Design review of the part shown in the three views and the two pictorial views. Dimensions are in mm from the part's minimum x, y and z. Give positions to 0.01 mm unless a question says otherwise; leave off trailing zeros. Order: outer loops, then holes, each group sorted by start corner. A loop starts at its lowest first (then second) coordinate and runs counter-clockwise, first axis right, second up.
Item 1: Consider section C-C (x = 4). Give the boundary of the cut face in (y, z).
Item 2: Consider section D-D (z = 12). Give the boundary of the cut face in (x, y).
Item 3: For P1, Ø7, axis at x = 4, z = 7.5, coming from the +Y side, flat-tipped, find the tip position at first contact; note if it passes through.
Item 4: Consider section A-A (y = 0.15). Give the number of separate pieces and of enclosed holes in the cut face, plus the area to 3 significant figures.
Item 5: Consider section B-B (x = 76.5). Give the boundary of the cut face in (y, z).
Item 6: For probe 1 along X at (y, z) = (0.25, 6.75); probe 2 along X at (y, z) = (0.4, 7.5); probe 3 along Z at (x, y) = (76.5, 0.35), list the stretches that pass through material, from the lowest coordinate up.
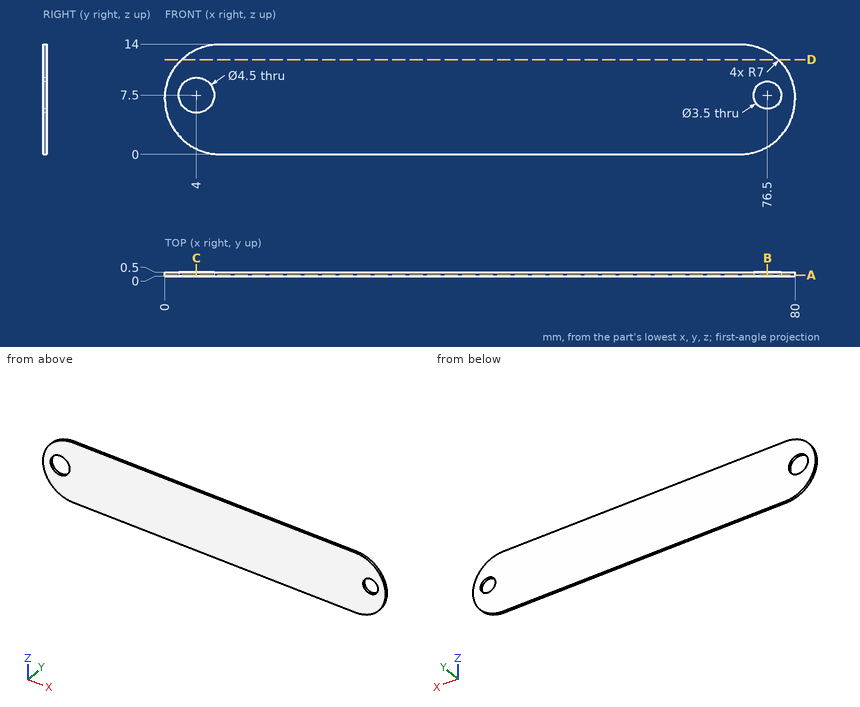
Resolved:
1. outline: (0, 0.68) - (0.5, 0.68) - (0.5, 5.25) - (0, 5.25) - close; (0, 9.75) - (0.5, 9.75) - (0.5, 13.32) - (0, 13.32) - close
2. outline: (2.1, 0) - (77.9, 0) - (77.9, 0.5) - (2.1, 0.5) - close
3. P1: stops at y = 0.5
4. separate pieces: 1
4. enclosed holes: 2
4. area: 1,050 mm2
5. outline: (0, 0.94) - (0.5, 0.94) - (0.5, 5.75) - (0, 5.75) - close; (0, 9.25) - (0.5, 9.25) - (0.5, 13.06) - (0, 13.06) - close
6. probe 1: x = 0 to 1.88, 6.12 to 74.92, 78.08 to 80
6. probe 2: x = 0.02 to 1.75, 6.25 to 74.75, 78.25 to 79.98
6. probe 3: z = 0.94 to 5.75, 9.25 to 13.06
